from build123d import *

# Parameters (mm, degrees)
ESQUISSE2_R                  = 1.5
ENL_V_MAT_EXTRU_1_DEPTH      = 83.632227369
ESQUISSE3_R                  = 1
ENL_V_MAT_EXTRU_2_DEPTH      = 3
R_P_TITION_CIRCULAIRE1_COUNT = 4
SKETCH1_R                    = 57.15
SKETCH1_R_2                  = 53.2
CUT_EXTRUDE1_DEPTH           = 88.2243372


with BuildPart() as part:
    # Esquisse1 → Base-Révolution (revolve)
    with BuildSketch(Plane(origin=(0, 0, 0), x_dir=(0, 0, -1), z_dir=(1, 0, 0)), mode=Mode.PRIVATE) as base_r_volution_sk:
        with BuildLine():
            Line((0, 25.5), (0, 26.3))
            Line((0, 26.3), (7.2, 26.3))
            ThreePointArc((7.2, 26.3), (14.271067812, 29.228932188), (17.2, 36.3))
            Line((17.2, 36.3), (17.2, 56))
            Line((17.2, 56), (22, 56))
            Line((22, 56), (22, 57.15))
            Line((22, 57.15), (32.8, 57.15))
            Line((32.8, 57.15), (32.8, 54.6))
            Line((32.8, 54.6), (27.8, 54.6))
            Line((27.8, 54.6), (27.8, 53.45))
            ThreePointArc((27.8, 53.45), (22.885607871, 51.414392129), (20.85, 46.5))
            Line((20.85, 46.5), (20.85, 36))
            ThreePointArc((20.85, 36), (17.774621202, 28.575378798), (10.35, 25.5))
            Line((10.35, 25.5), (1.5, 25.5))
            Line((1.5, 25.5), (0, 25.5))
        make_face()
    revolve(base_r_volution_sk.sketch.rotate(Axis((0, 0, 0), (0, 0, -1)), 90), axis=Axis((0, 0, 0), (0, 0, -1)))

    # Esquisse2 → Enlèv. mat.-Extru.1 (cut, through all)
    with BuildSketch(Plane.XY.offset(-17.2)):
        with Locations((0, 44.5)):
            Circle(ESQUISSE2_R)
        with Locations((18.099780617, 40.652772865)):
            Circle(ESQUISSE2_R)
        with Locations((33.069944734, 29.776311983)):
            Circle(ESQUISSE2_R)
        with Locations((42.322014975, 13.75125625)):
            Circle(ESQUISSE2_R)
        with Locations((44.256224344, -4.651516615)):
            Circle(ESQUISSE2_R)
        with Locations((38.538130468, -22.25)):
            Circle(ESQUISSE2_R)
        with Locations((26.156443727, -36.00125625)):
            Circle(ESQUISSE2_R)
        with Locations((9.252070241, -43.527568233)):
            Circle(ESQUISSE2_R)
        with Locations((-9.252070241, -43.527568233)):
            Circle(ESQUISSE2_R)
        with Locations((-26.156443727, -36.00125625)):
            Circle(ESQUISSE2_R)
        with Locations((-38.538130468, -22.25)):
            Circle(ESQUISSE2_R)
        with Locations((-44.256224344, -4.651516615)):
            Circle(ESQUISSE2_R)
        with Locations((-42.322014975, 13.75125625)):
            Circle(ESQUISSE2_R)
        with Locations((-33.069944734, 29.776311983)):
            Circle(ESQUISSE2_R)
        with Locations((-18.099780617, 40.652772865)):
            Circle(ESQUISSE2_R)
    extrude(amount=-ENL_V_MAT_EXTRU_1_DEPTH, mode=Mode.SUBTRACT)

    # Esquisse3 → Enlèv. mat.-Extru.2 (cut)
    with BuildSketch(Plane(origin=(0, 57.5, 0), x_dir=(-1, 0, 0), z_dir=(0, 1, 0))):
        with Locations(Location((0, -19.5, 0), (0, 0, 90))):
            Circle(ESQUISSE3_R)
    enl_v_mat_extru_2 = extrude(amount=-ENL_V_MAT_EXTRU_2_DEPTH, mode=Mode.SUBTRACT)

    # Répétition circulaire1: Enlèv. mat.-Extru.2 ×4 about axis
    r_p_tition_circulaire1_axis = Axis((0, 0, 0), (0, 0, 1))
    for i in range(1, R_P_TITION_CIRCULAIRE1_COUNT):
        add(enl_v_mat_extru_2.rotate(r_p_tition_circulaire1_axis, i * 360 / R_P_TITION_CIRCULAIRE1_COUNT), mode=Mode.SUBTRACT)

    # Sketch1 → Cut-Extrude1 (cut, through all)
    with BuildSketch(Plane(origin=(0, 0, -32.8), x_dir=(-1, 0, 0), z_dir=(0, 0, -1))):
        Circle(SKETCH1_R)
        Circle(SKETCH1_R_2, mode=Mode.SUBTRACT)
    extrude(amount=-CUT_EXTRUDE1_DEPTH, mode=Mode.SUBTRACT)


solid = part.part
Here's how the part is built. I have some questions about the finished solid (model axes, mm). A direction names the side the tool comes from. Coordinates: 2 decimals unless noted, no trailing zeros. Write each loop counter-clockwise with the first axis right and the second up, starting at its lowest first coordinate (ties: lowest second). Pieces come first, ordered by that corner, then holes.
1) If I drill on line 1 (Y direction, x = -3, z = -22.5); line 2 (Y direction, x = -1.5, z = -22); line 3 (Z direction, x = 23, y = 34), over which ranges is the centre line in solid material (lowest first)?
Filled in:
line 1: y = -53.12 to -50.91, 50.91 to 53.12
line 2: y = -53.18 to -50.31, 50.31 to 53.18
line 3: z = -20.85 to -17.2
2) If we section it at B-B (y = 0): List the corners of the cut face in (x, z) for me.
Filled in:
outline: (-53.2, -25.95) arc R6.95 cw to (-46.5, -20.85) - (-36, -20.85) arc R10.5 ccw to (-25.5, -10.35) - (-25.5, 0) - (-26.3, 0) - (-26.3, -7.2) arc R10 cw to (-36.3, -17.2) - (-53.2, -17.2) - close; (25.5, -10.35) arc R10.5 ccw to (36, -20.85) - (46.5, -20.85) arc R6.95 cw to (53.2, -25.95) - (53.2, -17.2) - (36.3, -17.2) arc R10 cw to (26.3, -7.2) - (26.3, 0) - (25.5, 0) - close
3) If we section it at C-C (z = -3.5): List the corners of the cut face in (x, y) for me, plus the area to 3 significant figures.
Filled in:
outline: circle Ø52.6 at (0, 0); hole circle Ø51 at (0, 0)
area: 130 mm2
4) If we section it at A-A (x = 0): List the corners of the cut face in (y, z) for me.
Filled in:
outline: (-53.2, -25.95) arc R6.95 cw to (-46.5, -20.85) - (-36, -20.85) arc R10.5 ccw to (-25.5, -10.35) - (-25.5, 0) - (-26.3, 0) - (-26.3, -7.2) arc R10 cw to (-36.3, -17.2) - (-53.2, -17.2) - close; (25.5, -10.35) arc R10.5 ccw to (36, -20.85) - (43, -20.85) - (43, -17.2) - (36.3, -17.2) arc R10 cw to (26.3, -7.2) - (26.3, 0) - (25.5, 0) - close; (46, -20.85) - (46.5, -20.85) arc R6.95 cw to (53.2, -25.95) - (53.2, -17.2) - (46, -17.2) - close
5) Which directions (+Z, -Z, +X, -X, +Y, -Y) give clear straight access to the entire face, cutting with the end or side of a thin tool? Please do faces 1 (the face through (23.9, 27.3, -20.85)), 2 (the face through (25.086, -7.9, -3.65)), 3 (the face through (-19.29, 39.74, -19)).
Filled in:
face 1: -Z
face 2: +Z
face 3: +Z, -Z
6) I'm going to push flat-ended pins straight in: pin 1 (3.5 mm diameter, centred on x = 9.25, y = -43.53, fed in from +Z); pin 2 (8 mm diameter, centred on x = 21.5, z = -17, fed in from -Y); pin 3 (2 mm diameter, centred on x = 26.5, y = -12.5, fed in from +Z). Where does each tip first touch, or does it pass through?
Filled in:
pin 1: stops at z = -17.2
pin 2: stops at y = -50.24
pin 3: stops at z = -13.2
7) If we section it at D-D (y = -22.25): Count the separate pieces of the cut face and the enclosed holes in it, plus the area to 3 significant figures.
Filled in:
separate pieces: 4
enclosed holes: 0
area: 302 mm2
8) Thinking about a two-plate mould opening in Y: for faces 4 (the face through (31.964, 30.79, -18.999)), 5 (the face through (-24.549, -47.198, -21.638)), 6 (the face through (-11, 35, -17.2)), which applies, +Y half, -Y half, draft (parallel to the pull), parting line (faces both ways), or undercut?
Filled in:
face 4: undercut
face 5: parting line
face 6: draft
